For this review, use the dimensioned drawing (mm, ordinates from the lowest corner) and the shaded views. A direction names the side the tool comes from. Coordinates: 2 decimals unless noted, no trailing zeros. Loops run counter-clockwise (first coordinate to the right, second up) from the corner with the lowest first, then second, coordinate; pieces in that order, holes last. Notation, with made-up numbers: (-6, 61.5) - (22, 61.5) arc R22 cw to (22, 85.5) - close; hole circle Ø11 at (-11, 81.25). An arc over 180 degrees is marked (long way). Return JSON: item names as keys, results as strings. Group by question number.
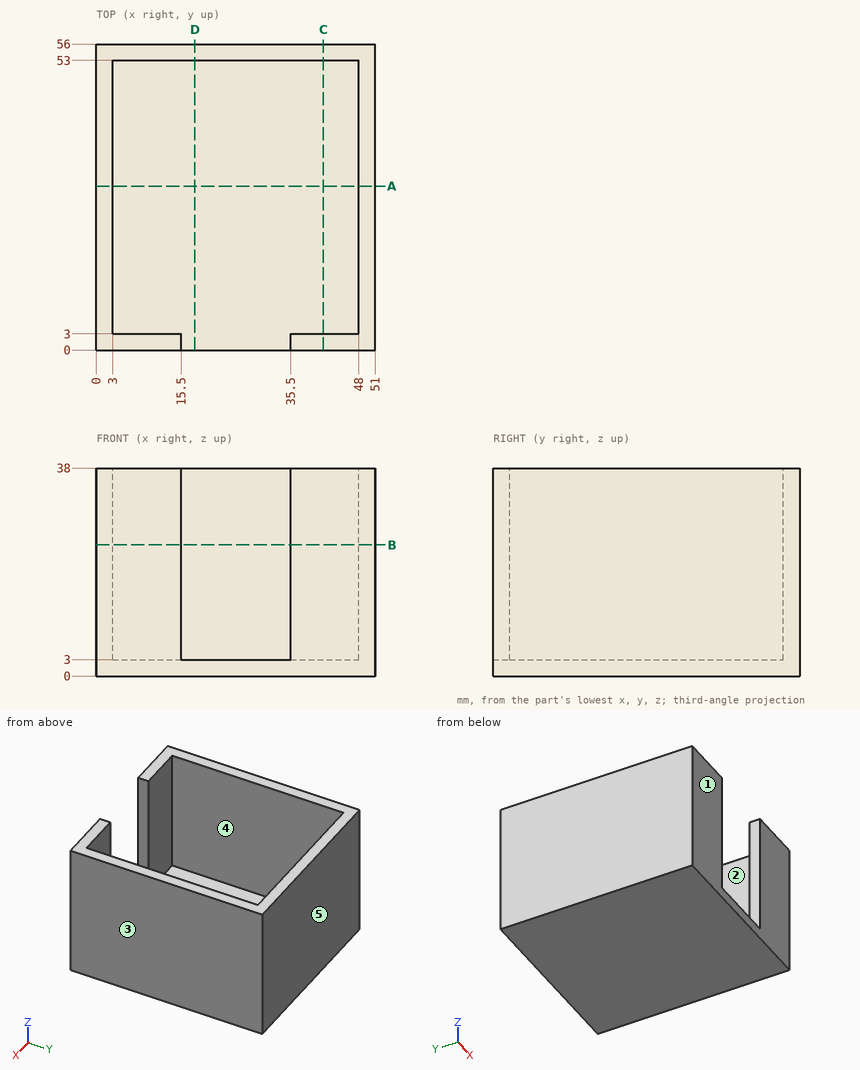
Item 1: To check wall thickness, follow line 1 (Y direction, x = 40.5, z = 35); line 2 (X direction, y = 33, z = 35); line 3 (Z direction, x = 6.5, y = 45). State the ranges of each line that lie inside material, in increasing order. Write a range as from..to.
Item 2: For the marked faces 1 and 2, list the 3-axis set-ups (+Z, -Z, +X, -X, +Y, -Y) from which the entire face can be reached by the end or side of a thin tool; tool diameter is ignored.
Item 3: Add section B-B (z = 24). State the section outline as (x, y) points.
Item 4: Draft analysis for pull direction Y (two halves, no side actions). For the marked faces 3, 4 and 5, state which applies: pulls with the +Y half, pulls with the -Y half, needs draft (parallel to the pull), parting line crosses it, or undercut.
Item 5: For P1, Ø22.5, axis at x = 26.5, y = 26, coming from the +Z side; P2, Ø2, axis at x = 42, y = 43.5, coming from the -Z side; P3, Ø3, axis at x = 26.5, z = 33.5, coming from the -Y side, all flat-tipped, find the tip position at first contact; note any pin that passes through.
Item 6: Add section C-C (x = 41.5). State the section outline as (y, z) points.
Item 7: Add section D-D (x = 18). State the section outline as (y, z) points.
Item 8: Add section A-A (y = 30). State the section outline as (x, z) points, then the cut area to 3 significant figures.
Answers below:
{
 "1": {"line 1": "y = 0..3, 53..56", "line 2": "x = 0..3, 48..51", "line 3": "z = 0..3"},
 "2": {"face 1": "+Z, -Z, +X, -X, -Y", "face 2": "+Z"},
 "3": {"outline": "(0, 0) - (15.5, 0) - (15.5, 3) - (3, 3) - (3, 53) - (48, 53) - (48, 3) - (35.5, 3) - (35.5, 0) - (51, 0) - (51, 56) - (0, 56) - close"},
 "4": {"face 3": "needs draft", "face 4": "undercut", "face 5": "pulls with the +Y half"},
 "5": {"P1": "stops at z = 3", "P2": "stops at z = 0", "P3": "stops at y = 53"},
 "6": {"outline": "(0, 0) - (56, 0) - (56, 38) - (53, 38) - (53, 3) - (3, 3) - (3, 38) - (0, 38) - close"},
 "7": {"outline": "(0, 0) - (56, 0) - (56, 38) - (53, 38) - (53, 3) - (0, 3) - close"},
 "8": {"outline": "(0, 0) - (51, 0) - (51, 38) - (48, 38) - (48, 3) - (3, 3) - (3, 38) - (0, 38) - close", "area": "363 mm^2"}
}
